Build history of the part. All positions in model axes, mm. Face numbers are marked on the shaded views. A direction names the side the tool comes from. Give positions to 0.01 mm unless a question says otherwise; leave off trailing zeros. Order: outer loops, then holes, each group sorted by start corner. A loop starts at its lowest first (then second) coordinate and runs counter-clockwise, first axis right, second up. Notation, with made-up numbers: M 52.5,68.25 L 58.5,68.25 A21 ccw 58.5,98.25 Z; hole C 8,62 d7. An arc over 180 degrees is marked long. One line per item, written item: value.
Autodesk Inventor part; units mm, degrees
ref_plane "YZ Plane" through (0, 0, 0) normal (1, 0, 0) x (0, 1, 0)
ref_plane "XZ Plane" through (0, 0, 0) normal (0, 1, 0) x (-1, 0, 0)
ref_plane "XY Plane" through (0, 0, 0) normal (0, 0, 1) x (1, 0, 0)
sketch "Sketch1" plane through (0, 0, 0) normal (0, 0, 1) x (1, 0, 0)
  line L0 (0, 0) -> (71, 0)
  line L1 (71, 0) -> (71, 72.4)
  line L2 (71, 72.4) -> (0, 72.4)
  line L3 (0, 72.4) -> (0, 0)
  dimension "d0" = 71
  dimension "d1" = 72.4
extrude "Extrusion1" add sketch "Sketch1" along normal blind 10
sketch "Sketch2" plane through (0, 0, 10) normal (0, 0, 1) x (1, 0, 0)
  line L0 (71, 0) -> (71, 72.4)
  line L1 (71, 12.4) -> (81, 12.4)
  line L2 (81, 12.4) -> (81, 52.4)
  line L3 (81, 52.4) -> (71, 52.4)
  line L4 (71, 52.4) -> (71, 12.4)
  line L5 (71, 72.4) -> (0, 72.4)
  circle A0 centre (76, 32.4) radius 2.5
  line L6 (0, 0) -> (71, 0)
  point P0 (81, 32.4)
  point P1 (76, 52.4)
  dimension "d4" = 10
  dimension "d5" = 40
  dimension "d7" = 5
  dimension "d53" = 20
extrude "Extrusion2" add sketch "Sketch2" against normal blind 10
sketch "Sketch3" plane through (0, 0, 10) normal (0, 0, 1) x (1, 0, 0)
  line L0 (71, 52.4) -> (81, 52.4)
  line L1 (71, 12.4) -> (81, 12.4)
  line L2 (81, 52.4) -> (71, 52.4)
  line L3 (71, 52.4) -> (71, 12.4)
  line L4 (71, 12.4) -> (81, 12.4)
  line L5 (81, 12.4) -> (81, 52.4)
  point P0 (0, 0)
extrude "Extrusion3" cut sketch "Sketch3" against normal blind 5
sketch "Sketch10" plane through (0, 0, 0) normal (0, 0, -1) x (-1, 0, 0)
  line L0 (0, 72.4) -> (0, 0)
  line L1 (0, 12.4) -> (10, 12.4)
  line L2 (10, 12.4) -> (10, 52.4)
  line L3 (10, 52.4) -> (0, 52.4)
  line L4 (0, 52.4) -> (0, 12.4)
  circle A0 centre (5, 32.4) radius 2.5
  point P0 (-81, 12.4)
  point P1 (10, 32.4)
  point P2 (5, 12.4)
  dimension "d40" = 10
  dimension "d41" = 40
  dimension "d42" = 5
extrude "Extrusion10" add sketch "Sketch10" against normal blind 5
sketch "Sketch11" plane through (0, 0, 0) normal (0, 0, -1) x (-1, 0, 0)
  line L0 (-71, 72.4) -> (0, 72.4)
  line L1 (-15.5, 72.4) -> (-55.5, 72.4)
  line L2 (-55.5, 72.4) -> (-55.5, 82.4)
  line L3 (-55.5, 82.4) -> (-15.5, 82.4)
  line L4 (-15.5, 82.4) -> (-15.5, 72.4)
  circle A0 centre (-35.5, 77.4) radius 2.5
  point P0 (0, 0)
  point P1 (-35.5, 82.4)
  point P2 (-35.5, 72.4)
  point P3 (-15.5, 77.4)
  dimension "d46" = 40
  dimension "d47" = 10
  dimension "d48" = 5
extrude "Extrusion11" add sketch "Sketch11" against normal blind 5
sketch "Sketch12" plane through (0, 0, 0) normal (0, 0, -1) x (-1, 0, 0)
  line L0 (0, 0) -> (-71, 0)
  line L1 (-55.5, 0) -> (-15.5, 0)
  line L2 (-15.5, 0) -> (-15.5, -10)
  line L3 (-15.5, -10) -> (-55.5, -10)
  line L4 (-55.5, -10) -> (-55.5, 0)
  circle A0 centre (-35.5, -5) radius 2.5
  point P0 (-55.5, 82.4)
  point P1 (-15.5, 82.4)
  point P2 (-35.5, -10)
  point P3 (-55.5, -5)
  dimension "d54" = 10
  dimension "d55" = 5
extrude "Extrusion12" add sketch "Sketch12" against normal blind 5
sketch "Sketch13" plane through (0, 0, 0) normal (0, 0, -1) x (-1, 0, 0)
  line L0 (-11, 22.7) -> (-60, 22.7)
  line L1 (-60, 22.7) -> (-60, 49.7)
  line L2 (-60, 49.7) -> (-11, 49.7)
  line L3 (-11, 49.7) -> (-11, 22.7)
  line L4 (0, 0) -> (-71, 0)
  line L5 (-71, 72.4) -> (0, 72.4)
  line L6 (-71, 0) -> (0, 0)
  line L7 (0, 0) -> (0, 72.4)
  line L8 (0, 72.4) -> (-71, 72.4)
  line L9 (-71, 72.4) -> (-71, 0)
  line L10 (-35.5, 56.1679) -> (-35.5, 16.2321) construction
  circle A0 centre (-35.5, 16.2321) radius 1.5
  circle A1 centre (-35.5, 56.1679) radius 1.5
  point P0 (-60, 36.2)
  point P1 (-71, 36.2)
  point P2 (-35.5, 49.7)
  point P3 (-35.5, 72.4)
  point P4 (-35.5, 36.2)
  dimension "d58" = 49
  dimension "d59" = 27
  dimension "d60" = 39.9357
  dimension "d61" = 3
  dimension "d62" = 3
extrude "Extrusion13" cut sketch "Sketch13" against normal through all contours L0 L1 L2 L3 | A0 | A1
properties part number "SP002" material "ABS Plastic"
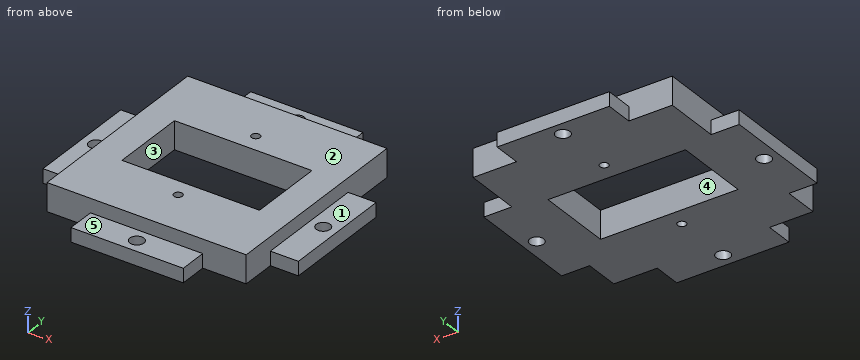
1) Mould opens along X. For the marked faces 4 and 5 say: released by +X, released by -X, zero draft, split by the parting line, or undercut.
Check values:
face 4: undercut
face 5: zero draft
2) Drill centre lines: probe 1 along Y at (x, z) = (35.5, 1.4); probe 2 along Y at (x, z) = (35.5, 7); probe 3 along Y at (x, z) = (27, 8). Where is each one in solid material? Low to high. Write a range as from..to.
Check values:
probe 1: -10..-7.5, -2.5..14.73, 17.73..22.7, 49.7..54.67, 57.67..74.9, 79.9..82.4
probe 2: 0..14.73, 17.73..22.7, 49.7..54.67, 57.67..72.4
probe 3: 0..22.7, 49.7..72.4
3) Tool access for the marked faces 1, 2 and 3: list every direction of +Z, -Z, +X, -X, +Y, -Y with a clear straight run to the whole face (end or side of a thin tool).
Check values:
face 1: +Z, +X, +Y, -Y
face 2: +Z, +X, -X, +Y, -Y
face 3: +Z, -Z
4) Saw through at B-B, the plane y = -5. Write the cut outline in (x, z).
Check values:
outline: M 15.5,0 L 33,0 L 33,5 L 15.5,5 Z; M 38,0 L 55.5,0 L 55.5,5 L 38,5 Z
5) Pin check, flat tips, straight feed: pin 1 (1.5 mm diameter, centred on x = -4.5, z = 2.5, fed in from +Y); pin 2 (5 mm diameter, centred on x = 37, y = -6.5, fed in from +Z); pin 3 (1 mm diameter, centred on x = 3.5, z = 5, fed in from +Y); pin 4 (4 mm diameter, centred on x = 76, y = 32.4, fed in from +Z). Stop position of each tip, or through.
Check values:
pin 1: y = 52.4
pin 2: z = 5
pin 3: y = 72.4
pin 4: through
6) Saw through at C-C, the plane y = 32.4. Write the cut outline in (x, z).
Check values:
outline: M -10,0 L -7.5,0 L -7.5,5 L -10,5 Z; M -2.5,0 L 11,0 L 11,10 L 0,10 L 0,5 L -2.5,5 Z; M 60,0 L 73.5,0 L 73.5,5 L 71,5 L 71,10 L 60,10 Z; M 78.5,0 L 81,0 L 81,5 L 78.5,5 Z
7) Saw through at D-D, the plane x = 35.5. Write the cut outline in (y, z), then the cut area to 3 significant figures.
Check values:
outline: M -10,0 L -7.5,0 L -7.5,5 L -10,5 Z; M -2.5,0 L 14.73,0 L 14.73,10 L 0,10 L 0,5 L -2.5,5 Z; M 17.73,0 L 22.7,0 L 22.7,10 L 17.73,10 Z; M 49.7,0 L 54.67,0 L 54.67,10 L 49.7,10 Z; M 57.67,0 L 74.9,0 L 74.9,5 L 72.4,5 L 72.4,10 L 57.67,10 Z; M 79.9,0 L 82.4,0 L 82.4,5 L 79.9,5 Z
area: 444 mm^2
8) Saw through at A-A, the plane x = 76. Write the cut outline in (y, z).
Check values:
outline: M 12.4,0 L 29.9,0 L 29.9,5 L 12.4,5 Z; M 34.9,0 L 52.4,0 L 52.4,5 L 34.9,5 Z
